Geometry: see drawing. Coordinates: mm, zero at the bounding-box minimum. Give positions to 0.01 mm unless a question says otherwise; leave off trailing zeros. Order: outer loops, then holes, each group sorted by start corner. A loop starts at its lowest first (then second) coordinate and runs counter-clockwise, first axis right, second up. Notation, with made-up numbers: (33, -27.5) - (80, -27.5) arc R32 cw to (80, 10.5) - close; hole circle Ø9 at (-16.5, 59). An arc over 180 degrees is marked (long way). Put each result on its own line as item: value. Start each with the question number.
1. Section A-A on z = 100. Return the cut outline in (x, y), plus the area to 3 significant figures.
2. Section B-B on x = 100. Return the cut outline in (y, z), plus the area to 3 significant figures.
3. First-contact query: P1, Ø14, axis at x = 100, z = 100, coming from the +Y side; P2, Ø1.5, axis at x = 393, z = 101.5, coming from the -Y side. Flat tips, straight axial feed; report the tip coordinate or a pass-through.
4. Ray query, line 1 along X through (y, z) = (4.5, 100); line 2 along X through (y, z) = (7.75, 97); line 3 along Z through (x, y) = (540, 7). Return the intervals inside material, ascending. Write a range as from..to.
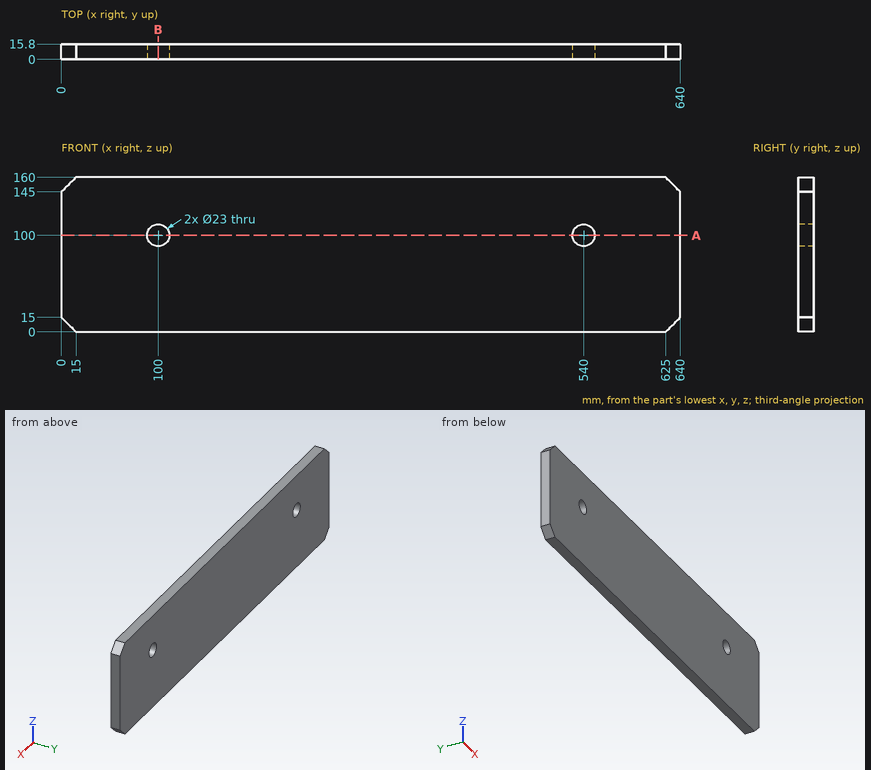
Resolved:
1. outline: (0, 0) - (88.5, 0) - (88.5, 15.8) - (0, 15.8) - close; (111.5, 0) - (528.5, 0) - (528.5, 15.8) - (111.5, 15.8) - close; (551.5, 0) - (640, 0) - (640, 15.8) - (551.5, 15.8) - close
1. area: 9,390 mm^2
2. outline: (0, 0) - (15.8, 0) - (15.8, 88.5) - (0, 88.5) - close; (0, 111.5) - (15.8, 111.5) - (15.8, 160) - (0, 160) - close
2. area: 2,160 mm^2
3. P1: through
3. P2: y = 0
4. line 1: 0..88.5, 111.5..528.5, 551.5..640
4. line 2: 0..88.9, 111.1..528.9, 551.1..640
4. line 3: 0..88.5, 111.5..160
